Design review of the part built by this model. Coordinates are the model's own, in mm. Face numbers are marked on the shaded views. Coordinates: 2 decimals unless noted, no trailing zeros. Loops run counter-clockwise (first coordinate to the right, second up) from the corner with the lowest first, then second, coordinate; pieces in that order, holes last. Notation, with made-up numbers: (15.5, 1.25) -> (29.5, 1.25) arc R20 cw to (29.5, 8.25) -> close; hole circle Ø4 at (65.5, 88). An arc over 180 degrees is marked (long way). Use a Markdown table: item, result. Add a question column.
Q1. Take a section at A-A on x = 0. Write out the cut boundary in (y, z), plus the area to 3 significant figures.
Q2. Draft analysis for pull direction Y (two halves, no side actions). For the marked faces 1, 2 and 3, state which applies: pulls with the +Y half, pulls with the -Y half, needs draft (parallel to the pull), parting line crosses it, or undercut.
Q3. Take a section at D-D on x = 11.5. Write out the cut boundary in (y, z).
Q4. Clearance check with flat-ended pins moving along their axes: pin 1 Ø3.5 at (x, y) = (-0.5, 10) entering from -Z; pin 2 Ø8 at (x, z) = (-9, -21.5) entering from +Y; pin 3 Ø4 at (x, z) = (-5, -8.5) entering from +Y. State where each tip first meets the part, or that it passes through.
Q5. Take a section at C-C on z = -24. Write out the cut boundary in (x, y), plus the area to 3 significant figures.
Q6. For probe 1 along Z at (x, y) = (0, 0.8); probe 2 along X at (y, z) = (1.4, -24); probe 3 along Y at (x, z) = (12.5, -9), list the stretches that pass through material, from the lowest coordinate up.
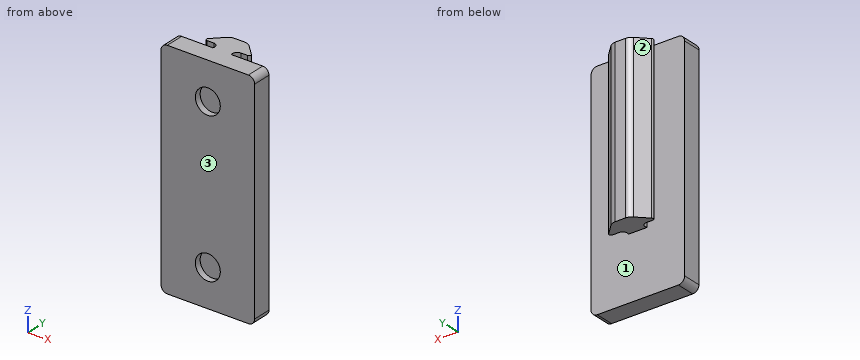
from build123d import *

# Parameters (mm, degrees)
BOSS_EXTRUDE1_DEPTH      = 6
SKETCH2_R                = 4
CUT_EXTRUDE1_DEPTH       = 2
SKETCH3_W                = 6
SKETCH3_H                = 1.2
BOSS_EXTRUDE2_DEPTH      = 36
BOSS_EXTRUDE2_DEPTH_BACK = 16


with BuildPart() as part:
    # Sketch1 → Boss-Extrude1 (new body)
    with BuildSketch(Plane(origin=(0, 0, 0), x_dir=(1, 0, 0), z_dir=(0, 1, 0))):
        with BuildLine():
            Line((-13, 36), (13, 36))
            ThreePointArc((13, 36), (14.414213562, 35.414213562), (15, 34))
            Line((15, 34), (15, -34))
            ThreePointArc((15, -34), (14.414213562, -35.414213562), (13, -36))
            Line((13, -36), (-13, -36))
            ThreePointArc((-13, -36), (-14.414213562, -35.414213562), (-15, -34))
            Line((-15, -34), (-15, 34))
            ThreePointArc((-15, 34), (-14.414213562, 35.414213562), (-13, 36))
        make_face()
    extrude(amount=BOSS_EXTRUDE1_DEPTH)

    # Sketch2 → Cut-Extrude1 (cut)
    with BuildSketch(Plane(origin=(0, 0, 0), x_dir=(1, 0, 0), z_dir=(0, 1, 0))):
        with Locations((0, 24)):
            Circle(SKETCH2_R)
        with Locations((0, -24)):
            Circle(SKETCH2_R)
    extrude(amount=CUT_EXTRUDE1_DEPTH, mode=Mode.SUBTRACT)

    # Sketch3 → Boss-Extrude2 (add, two sides)
    with BuildSketch(Plane.XY) as boss_extrude2_sk:
        with BuildLine():
            Line((-4.343002999, 5.144651552), (-4.916686599, 5.144651552))
            Line((-4.916686599, 5.144651552), (-4.916686599, 3.944651552))
            Line((-4.916686599, 3.944651552), (4.917480601, 3.944651552))
            Line((4.917480601, 3.944651552), (4.917480601, 5.144651552))
            Line((4.917480601, 5.144651552), (4.343796972, 5.144651552))
            ThreePointArc((4.343796972, 5.144651552), (2.838896972, 6.649551552), (4.343796972, 8.154451552))
            Line((4.343796972, 8.154451552), (6.475191456, 8.154451552))
            ThreePointArc((6.475191456, 8.154451552), (7.044301248, 8.534718558), (6.910769234, 9.206029329))
            Line((6.910769234, 9.206029329), (3.580725693, 12.53607287))
            ThreePointArc((3.580725693, 12.53607287), (2.6804509, 13.137617255), (1.618504375, 13.348851552))
            Line((1.618504375, 13.348851552), (-1.617710374, 13.348851552))
            ThreePointArc((-1.617710374, 13.348851552), (-2.679656898, 13.137617255), (-3.579931691, 12.53607287))
            Line((-3.579931691, 12.53607287), (-6.909975232, 9.206029329))
            ThreePointArc((-6.909975232, 9.206029329), (-7.043507247, 8.534718558), (-6.474397455, 8.154451552))
            Line((-6.474397455, 8.154451552), (-4.343002999, 8.154451552))
            ThreePointArc((-4.343002999, 8.154451552), (-2.838102999, 6.649551552), (-4.343002999, 5.144651552))
        make_face()
        with Locations((-7.916686599, 4.544651552)):
            Rectangle(SKETCH3_W, SKETCH3_H)
        with Locations((7.917480601, 4.544651552)):
            Rectangle(SKETCH3_W, SKETCH3_H)
    extrude(amount=BOSS_EXTRUDE2_DEPTH)
    extrude(boss_extrude2_sk.sketch, amount=-BOSS_EXTRUDE2_DEPTH_BACK)


solid = part.part
Answer list:
| question | item | result |
|---|---|---|
| 1 | outline | (0, -36) -> (6, -36) -> (6, -16) -> (13.35, -16) -> (13.35, 36) -> (0, 36) -> (0, 28) -> (2, 28) -> (2, 20) -> (0, 20) -> (0, -20) -> (2, -20) -> (2, -28) -> (0, -28) -> close |
| 1 | area | 782 mm² |
| 2 | face 1 | undercut |
| 2 | face 2 | pulls with the +Y half |
| 2 | face 3 | pulls with the -Y half |
| 3 | outline | (0, -36) -> (6, -36) -> (6, 36) -> (0, 36) -> close |
| 4 | pin 1 | z = -16 |
| 4 | pin 2 | y = 6 |
| 4 | pin 3 | y = 12.98 |
| 5 | outline | (-15, 0) -> (-4, 0) -> (-4, 2) -> (4, 2) -> (4, 0) -> (15, 0) -> (15, 6) -> (-15, 6) -> close |
| 5 | area | 164 mm² |
| 6 | probe 1 | -36 to -28, -20 to 20, 28 to 36 |
| 6 | probe 2 | -15 to -4, 4 to 15 |
| 6 | probe 3 | 0 to 6 |
